Verification items for the finished model (mm, model axes). Face numbers are marked on the shaded views. A direction names the side the tool comes from. Round coordinates to 2 decimals unless told otherwise and drop trailing zeros. Write each loop counter-clockwise with the first axis right and the second up, starting at its lowest first coordinate (ties: lowest second). Pieces come first, ordered by that corner, then holes.
from build123d import *

# Parameters (mm, degrees)
F1_DEPTH  = 25
F3_DEPTH  = 20
F4_R      = 3.5
F5_DEPTH  = 5
F6_R      = 5
F6_R_2    = 1.4
F7_DEPTH  = 8
F8_R      = 2.75
F9_DEPTH  = 10
F10_R     = 4.25
F11_DEPTH = 5
F12_R     = 2.75
F13_DEPTH = 10
F14_R     = 4.25
F15_DEPTH = 5
F16_R     = 2.75
F17_DEPTH = 25


with BuildPart() as f1:
    # F0 (on Front) → F1 (new body)
    with BuildSketch(Plane.XZ):
        Polygon((200, 0), (0, 0), (0, -100), (172, -100), (172, -94.5), (176.5, -94.5), (194.5, -76.5), (194.5, -72), (200, -72), align=None)
    extrude(amount=F1_DEPTH)

    # F2 (on face) → F3 (cut)
    with BuildSketch(Plane.XZ.offset(25)):
        Polygon((190, -7.5), (15, -7.5), (15, -90), (165.893398, -90), (190, -65.893398), align=None)
    extrude(amount=-F3_DEPTH, mode=Mode.SUBTRACT)

    # F4 (on face) → F5 (cut, through all)
    with BuildSketch(Plane.XZ.offset(5)):
        Polygon((155, -12.5), (77, -12.5), (77, -26.5), (32, -26.5), (32, -56.5), (77, -56.5), (77, -63.5), (155, -63.5), align=None)
        with Locations((153, -82.25)):
            Circle(F4_R)
        with Locations((118.5, -82.25)):
            Circle(F4_R)
        with BuildLine():
            Line((133, -82.25), (133, -77.25))
            ThreePointArc((133, -77.25), (132, -76.25), (131, -77.25))
            Line((131, -77.25), (131, -82.25))
            Line((131, -82.25), (131, -87.25))
            ThreePointArc((131, -87.25), (132, -88.25), (133, -87.25))
            Line((133, -87.25), (133, -82.25))
        make_face()
        with BuildLine():
            ThreePointArc((137, -77.25), (136, -76.25), (135, -77.25))
            Line((135, -77.25), (135, -82.25))
            Line((135, -82.25), (135, -87.25))
            ThreePointArc((135, -87.25), (136, -88.25), (137, -87.25))
            Line((137, -87.25), (137, -82.25))
            Line((137, -82.25), (137, -77.25))
        make_face()
        with BuildLine():
            ThreePointArc((141, -77.25), (140, -76.25), (139, -77.25))
            Line((139, -77.25), (139, -82.25))
            Line((139, -82.25), (139, -87.25))
            ThreePointArc((139, -87.25), (140, -88.25), (141, -87.25))
            Line((141, -87.25), (141, -82.25))
            Line((141, -82.25), (141, -77.25))
        make_face()
        with Locations((77.5, -79.25)):
            Circle(F4_R)
    extrude(amount=-F5_DEPTH, mode=Mode.SUBTRACT)

    # F6 (on face) → F7 (join)
    with BuildSketch(Plane(origin=(0, 0, 0), x_dir=(-1, 0, 0), z_dir=(0, 1, 0))):
        with Locations((-69, -6)):
            Circle(F6_R)
        with Locations((-69, -6)):
            Circle(F6_R_2, mode=Mode.SUBTRACT)
        with Locations((-162, -6)):
            Circle(F6_R)
        with Locations((-162, -6)):
            Circle(F6_R_2, mode=Mode.SUBTRACT)
        with Locations((-162, -71)):
            Circle(F6_R)
        with Locations((-162, -71)):
            Circle(F6_R_2, mode=Mode.SUBTRACT)
        with Locations((-69, -71)):
            Circle(F6_R)
        with Locations((-69, -71)):
            Circle(F6_R_2, mode=Mode.SUBTRACT)
    extrude(amount=F7_DEPTH)

    # F8 (on face) → F9 (cut, through all)
    with BuildSketch(Plane(origin=(190, 0, 0), x_dir=(0, -1, 0), z_dir=(-1, 0, 0))):
        with Locations((15, -36.696699)):
            Circle(F8_R)
    extrude(amount=-F9_DEPTH, mode=Mode.SUBTRACT)

    # F10 (on face) → F11 (cut)
    with BuildSketch(Plane(origin=(190, 0, 0), x_dir=(0, -1, 0), z_dir=(-1, 0, 0))):
        with Locations((15, -36.696699)):
            Circle(F10_R)
    extrude(amount=-F11_DEPTH, mode=Mode.SUBTRACT)

    # F12 (on face) → F13 (cut, through all)
    with BuildSketch(Plane.XY.offset(-90)):
        with Locations((30, -15)):
            Circle(F12_R)
        with Locations((155.893398, -15)):
            Circle(F12_R)
    extrude(amount=-F13_DEPTH, mode=Mode.SUBTRACT)

    # F14 (on face) → F15 (cut)
    with BuildSketch(Plane.XY.offset(-90)):
        with Locations((30, -15)):
            Circle(F14_R)
        with Locations((155.893398, -15)):
            Circle(F14_R)
    extrude(amount=-F15_DEPTH, mode=Mode.SUBTRACT)

    # F16 (on face) → F17 (cut, through all)
    with BuildSketch(Plane.XZ.offset(25)):
        with Locations((7.5, -20)):
            Circle(F16_R)
        with Locations((7.5, -80)):
            Circle(F16_R)
    extrude(amount=-F17_DEPTH, mode=Mode.SUBTRACT)


solid = f1.part
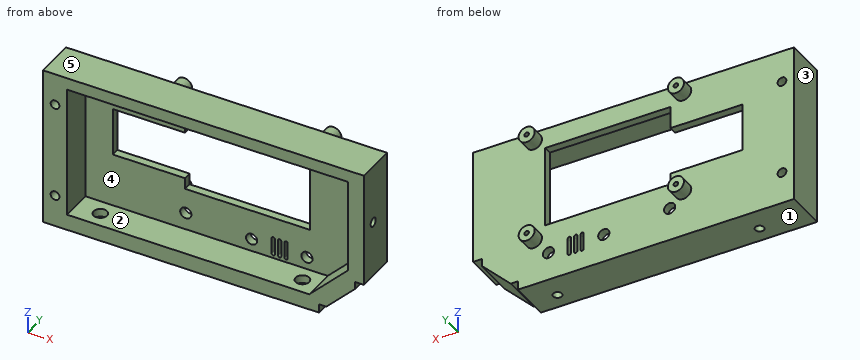
Q1. Depth check by flat-ended pin: P1, Ø1.6, axis at x = 197, y = -15, coming from the -Z side; P2, Ø2.5, axis at y = -2.5, z = -81.5, coming from the +X side; P3, Ø4, axis at x = 58, z = -14.5, coming from the +Y side. Enter the tip coordinate at first touch or a pass-through.
Recorded:
P1: stops at z = -72
P2: stops at x = 190.75
P3: stops at y = 0
Q2. Tool access check on the marked faces 1 and 2. Record the directions out of +Z, -Z, +X, -X, +Y, -Y that give a thin tool (end or side, any length) a straight path to the whole face; none if there is none.
Recorded:
face 1: -Z, +X, -X, +Y, -Y
face 2: -Y
Q3. Sectioned sample at C-C (z = -48). Enter the section's corners in (x, y), plus the area to 3 significant figures.
Recorded:
outline: (0, -25) - (15, -25) - (15, -5) - (32, -5) - (32, 0) - (0, 0) - close; (155, -5) - (190, -5) - (190, -25) - (200, -25) - (200, 0) - (155, 0) - close
area: 885 mm2
Q4. Material ranges on line 1 along Z through (x, y) = (76.5, -0.5); line 2 along X through (y, z) = (-2, -26); line 3 along Z through (x, y) = (165.5, -11), recorded low to high.
Recorded:
line 1: z = -100 to -82.6, -75.9 to -56.5, -26.5 to 0
line 2: x = 0 to 77, 155 to 200
line 3: z = -100 to -90, -7.5 to 0
Q5. Release check for a two-part mould opening along X. For the marked faces 3, 4 and 5 record: released by +X, released by -X, zero draft, split by the parting line, or undercut.
Recorded:
face 3: released by -X
face 4: undercut
face 5: zero draft
Q6. Sectioned sample at A-A (y = -8). Enter the section's corners in (x, z).
Recorded:
outline: (0, -100) - (172, -100) - (172, -94.5) - (176.5, -94.5) - (194.5, -76.5) - (194.5, -72) - (200, -72) - (200, 0) - (0, 0) - close; hole circle Ø5.5 at (7.5, -80); hole circle Ø5.5 at (7.5, -20); hole (15, -90) - (165.89, -90) - (190, -65.89) - (190, -7.5) - (15, -7.5) - close
Q7. Sectioned sample at B-B (x = 94.5). Enter the section's corners in (y, z).
Recorded:
outline: (-25, -100) - (0, -100) - (0, -63.5) - (-5, -63.5) - (-5, -90) - (-25, -90) - close; (-25, -7.5) - (-5, -7.5) - (-5, -12.5) - (0, -12.5) - (0, 0) - (-25, 0) - close
